Part model, mm, in its own coordinate system. A direction names the side the tool comes from. Give positions to 0.01 mm unless a question says otherwise; leave off trailing zeros. Write each loop counter-clockwise with the first axis right and the second up, starting at its lowest first coordinate (ties: lowest second). Pieces come first, ordered by that corner, then holes. Notation, with made-up numbers: M 70,75.25 L 123,75.25 A18 cw 123,108.25 Z; hole C -15,-2 d10. An arc over 180 degrees is marked long. Use CSV: the item, a comma, the result in double quotes. Start each with the question number.
Item 1: Which spindle directions (+Z, -Z, +X, -X, +Y, -Y) get a long thin tool onto all of the face, cutting with end or side? Do faces 4 (the flat face through (2, 3, 6)), 5 (the flat face through (13, 2, -11.075)), 6 (the flat face through (-17, -1, -4.231)), 7 (the flat face through (-11, -3.5, 6)), 8 (the flat face through (-15.107, -2, 6)). Say none if no direction does.
Item 2: Cut at A-A (y = -1.5). List the corners of the cut face in (x, z), then the cut area to 3 significant figures.
Item 3: Drill centre lines: line 1 (Y direction, x = -12, z = -16); line 2 (X direction, y = 2.5, z = 15.5); line 3 (Z direction, x = -10, y = 2.25). Where is each one in solid material? Low to high. Write a range as [from, to].
Item 4: Mould opens along X. For faces 1 (the cylindrical face through (2.087, 2.098, -30.076)), 2 (the flat face through (7, 2.4, -26)), 3 (the cylindrical face through (-23.35, 2.1, 5.62)) say: released by +X, released by -X, zero draft, split by the parting line, or undercut.
Item 5: Pin check, flat tips, straight feed: pin 1 (1.7 mm diameter, centred on x = -2.5, z = 37.5, fed in from +Y); pin 2 (1.2 mm diameter, centred on x = 12, y = 2, fed in from +Z); pin 3 (1 mm diameter, centred on x = 22, z = -21, fed in from -Y); pin 4 (1.8 mm diameter, centred on x = 8.29, z = -25.93, fed in from -Y). Stop position of each tip, or through.
from build123d import *

# Parameters (mm, degrees)
BOSS_EXTRUDE1_DEPTH = 3
CUT_EXTRUDE1_DEPTH  = 1
FILLET1_R           = 3
SKETCH6_W           = 12
SKETCH6_H           = 20.5
BOSS_EXTRUDE3_DEPTH = 4.5
SKETCH28_W          = 0.3
SKETCH28_H          = 20.5
CUT_EXTRUDE18_DEPTH = 4.5
SKETCH44_R          = 1.1
CUT_EXTRUDE26_DEPTH = 10
SKETCH45_R          = 1.1
CUT_EXTRUDE27_DEPTH = 10
SKETCH47_R          = 1.7
CUT_EXTRUDE29_DEPTH = 0.6
SKETCH13_W          = 3
SKETCH13_H          = 20.5
CUT_EXTRUDE30_DEPTH = 3
SKETCH49_W          = 6.485663297
SKETCH49_H          = 3.694682329
CUT_EXTRUDE31_DEPTH = 8
SKETCH48_R          = 0.75
SKETCH48_W          = 4.647178446
SKETCH48_H          = 1.5
CUT_EXTRUDE33_DEPTH = 8
FILLET2_R           = 0.5
BOSS_EXTRUDE4_DEPTH = 1


with BuildPart() as part:
    # Sketch1 → Boss-Extrude1 (new body)
    with BuildSketch(Plane(origin=(0, 0, 0), x_dir=(1, 0, 0), z_dir=(0, 1, 0))):
        with BuildLine():
            Line((-19.206896552, 30.931034483), (22.793103448, 30.931034483))
            ThreePointArc((22.793103448, 30.931034483), (26.328637354, 29.466568389), (27.793103448, 25.931034483))
            Line((27.793103448, 25.931034483), (27.793103448, -38.068965517))
            ThreePointArc((27.793103448, -38.068965517), (26.328637354, -41.604499423), (22.793103448, -43.068965517))
            Line((22.793103448, -43.068965517), (-19.206896552, -43.068965517))
            ThreePointArc((-19.206896552, -43.068965517), (-22.742430458, -41.604499423), (-24.206896552, -38.068965517))
            Line((-24.206896552, -38.068965517), (-24.206896552, 25.931034483))
            ThreePointArc((-24.206896552, 25.931034483), (-22.742430458, 29.466568389), (-19.206896552, 30.931034483))
        make_face()
    extrude(amount=BOSS_EXTRUDE1_DEPTH)

    # Sketch3 → Cut-Extrude1 (cut)
    with BuildSketch(Plane(origin=(0, 0, 0), x_dir=(-1, 0, 0), z_dir=(0, -1, 0))):
        with BuildLine():
            Line((18.206896552, 29.931034483), (-21.793103448, 29.931034483))
            ThreePointArc((-21.793103448, 29.931034483), (-25.328637354, 28.466568389), (-26.793103448, 24.931034483))
            Line((-26.793103448, 24.931034483), (-26.793103448, -37.068965517))
            ThreePointArc((-26.793103448, -37.068965517), (-25.328637354, -40.604499423), (-21.793103448, -42.068965517))
            Line((-21.793103448, -42.068965517), (18.206896552, -42.068965517))
            ThreePointArc((18.206896552, -42.068965517), (21.742430458, -40.604499423), (23.206896552, -37.068965517))
            Line((23.206896552, -37.068965517), (23.206896552, 24.931034483))
            ThreePointArc((23.206896552, 24.931034483), (21.742430458, 28.466568389), (18.206896552, 29.931034483))
        make_face()
    extrude(amount=-CUT_EXTRUDE1_DEPTH, mode=Mode.SUBTRACT)

    # Fillet1
    fillet1_edges = [part.edges().sort_by_distance(p)[0] for p in [
        (-22.742430458, 3, -29.466568389),
        (1.793103448, 3, -30.931034483),
        (26.328637354, 3, -29.466568389),
        (27.793103448, 3, 6.068965517),
        (26.328637354, 3, 41.604499423),
        (1.793103448, 3, 43.068965517),
        (-22.742430458, 3, 41.604499423),
        (-24.206896552, 3, 6.068965517),
    ]]
    fillet(fillet1_edges, radius=FILLET1_R - 0.0001)  # a hair under: the kernel refuses the full size

    # Sketch6 → Boss-Extrude3 (add)
    with BuildSketch(Plane.XZ.offset(-1)):
        with Locations((-16.606896552, 6.018965517)):
            Rectangle(SKETCH6_W, SKETCH6_H)
    extrude(amount=BOSS_EXTRUDE3_DEPTH)

    # Sketch28 → Cut-Extrude18 (cut)
    with BuildSketch(Plane.XZ.offset(3.5)):
        with Locations((-22.456896552, 6.018965517)):
            Rectangle(SKETCH28_W, SKETCH28_H)
    extrude(amount=-CUT_EXTRUDE18_DEPTH, mode=Mode.SUBTRACT)

    # Sketch44 → Cut-Extrude26 (cut)
    with BuildSketch(Plane.XZ.offset(-1)):
        with Locations(Location((-2.026896552, 38.068965517, 0), (0, 0, 270))):
            Circle(SKETCH44_R)
    extrude(amount=-CUT_EXTRUDE26_DEPTH, mode=Mode.SUBTRACT)

    # Sketch45 → Cut-Extrude27 (cut)
    with BuildSketch(Plane.XZ.offset(-1)):
        with Locations(Location((8.293103448, -25.931034483, 0), (0, 0, 270))):
            Circle(SKETCH45_R)
    extrude(amount=-CUT_EXTRUDE27_DEPTH, mode=Mode.SUBTRACT)

    # Sketch47 → Cut-Extrude29 (cut)
    with BuildSketch(Plane(origin=(0, 3, 0), x_dir=(1, 0, 0), z_dir=(0, 1, 0))):
        with Locations(Location((8.293103448, 25.931034483, 0), (0, 0, 270))):
            Circle(SKETCH47_R)
        with Locations(Location((-2.026896552, -38.068965517, 0), (0, 0, 270))):
            Circle(SKETCH47_R)
    extrude(amount=-CUT_EXTRUDE29_DEPTH, mode=Mode.SUBTRACT)

    # Sketch13 → Cut-Extrude30 (cut)
    with BuildSketch(Plane.XZ.offset(3.5)):
        with Locations((-13.606896552, 6.018965517)):
            Rectangle(SKETCH13_W, SKETCH13_H)
    extrude(amount=-CUT_EXTRUDE30_DEPTH, mode=Mode.SUBTRACT)

    # Sketch49 → Cut-Extrude31 (cut)
    with BuildSketch(Plane(origin=(0, 3, 0), x_dir=(1, 0, 0), z_dir=(0, 1, 0))):
        with Locations((13.444488672, 12.922014382)):
            Rectangle(SKETCH49_W, SKETCH49_H)
    extrude(amount=-CUT_EXTRUDE31_DEPTH, mode=Mode.SUBTRACT)

    # Sketch48 → Cut-Extrude33 (cut)
    with BuildSketch(Plane(origin=(0, 3, 0), x_dir=(1, 0, 0), z_dir=(0, 1, 0))):
        with Locations(Location((13.919849349, -5.418160984, 0), (0, 0, 270))):
            Circle(SKETCH48_R)
        with Locations((15.692920165, -0.222236134)):
            Rectangle(SKETCH48_W, SKETCH48_H)
    extrude(amount=-CUT_EXTRUDE33_DEPTH, mode=Mode.SUBTRACT)

    # Fillet2
    fillet2_edges = [part.edges().sort_by_distance(p)[0] for p in [
        (10.201657023, 3, -12.922014382),
        (13.444488671, 3, -11.074673217),
        (16.68732032, 3, -12.922014382),
        (13.444488671, 3, -14.769355546),
        (13.369330942, 3, 0.222236134),
        (15.692920165, 3, 0.972236134),
        (18.016509388, 3, 0.222236134),
        (15.692920165, 3, -0.527763866),
        (13.919849349, 3, 4.668160984),
    ]]
    fillet(fillet2_edges, radius=FILLET2_R)

    # Sketch51 → Boss-Extrude4 (add)
    with BuildSketch(Plane(origin=(0, 0, 0), x_dir=(1, 0, 0), z_dir=(0, 1, 0))):
        with BuildLine():
            Line((26.793103448, 24.931034483), (26.793103448, -37.068965517))
            ThreePointArc((26.793103448, -37.068965517), (25.328637354, -40.604499423), (21.793103448, -42.068965517))
            Line((21.793103448, -42.068965517), (-18.206896552, -42.068965517))
            ThreePointArc((-18.206896552, -42.068965517), (-21.742430458, -40.604499423), (-23.206896552, -37.068965517))
            Line((-23.206896552, -37.068965517), (-23.206896552, 24.931034483))
            ThreePointArc((-23.206896552, 24.931034483), (-21.742430458, 28.466568389), (-18.206896552, 29.931034483))
            Line((-18.206896552, 29.931034483), (21.793103448, 29.931034483))
            ThreePointArc((21.793103448, 29.931034483), (25.328637354, 28.466568389), (26.793103448, 24.931034483))
        make_face()
        with BuildLine():
            Line((21.793103448, -41.568965517), (-18.206896552, -41.568965517))
            ThreePointArc((-18.206896552, -41.568965517), (-21.388877067, -40.250946033), (-22.706896552, -37.068965517))
            Line((-22.706896552, -37.068965517), (-22.706896552, 24.931034483))
            ThreePointArc((-22.706896552, 24.931034483), (-21.388877067, 28.113014998), (-18.206896552, 29.431034483))
            Line((-18.206896552, 29.431034483), (21.793103448, 29.431034483))
            ThreePointArc((21.793103448, 29.431034483), (24.975083964, 28.113014998), (26.293103448, 24.931034483))
            Line((26.293103448, 24.931034483), (26.293103448, -37.068965517))
            ThreePointArc((26.293103448, -37.068965517), (24.975083964, -40.250946033), (21.793103448, -41.568965517))
        make_face(mode=Mode.SUBTRACT)
    extrude(amount=BOSS_EXTRUDE4_DEPTH)


solid = part.part
Worked answers:
1,face 4,"+Z, -Z, +X, -X, +Y"
1,face 5,"+Y, -Y"
1,face 6,"-Y"
1,face 7,"+Z, -Z, +X, -X, -Y"
1,face 8,"+Z, -Z, -Y"
2,outline,"M -22.31,-4.23 L -15.11,-4.23 L -15.11,16.27 L -22.31,16.27 Z; M -12.11,-4.23 L -10.61,-4.23 L -10.61,16.27 L -12.11,16.27 Z"
2,area,"178 mm^2"
3,line 1,"y = [1, 3]"
3,line 2,"x = [-22.87, 26.45]"
3,line 3,"z = [-29.92, 42.05]"
4,face 1,"zero draft"
4,face 2,"undercut"
4,face 3,"released by -X"
5,pin 1,"stops at y = 2.4"
5,pin 2,"stops at z = 42.72"
5,pin 3,"stops at y = 1"
5,pin 4,"passes through"
